from build123d import *

# Parameters (mm, degrees)
F0_W     = 63.5
F0_H     = 71.628
F1_DEPTH = 21.59
F2_W     = 36.83
F2_H     = 50.8
F3_DEPTH = 21.59
F5_DEPTH = 50.8
F6_R     = 3.937
F7_DEPTH = 43.181


with BuildPart() as f1:
    # F0 (on Top) → F1 (new body)
    with BuildSketch(Plane.XY):
        with Locations((31.75, 35.814)):
            Rectangle(F0_W, F0_H)
    extrude(amount=-F1_DEPTH)

    # F2 (on face) → F3 (join)
    with BuildSketch(Plane.XY):
        with Locations((28.575, 46.228)):
            Rectangle(F2_W, F2_H)
    extrude(amount=F3_DEPTH)

    # F4 (on face) → F5 (cut)
    with BuildSketch(Plane.XZ.offset(-20.828)):
        Polygon((10.16, 0), (16.51, 21.59), (10.16, 21.59), align=None)
    extrude(amount=-F5_DEPTH, mode=Mode.SUBTRACT)

    # F6 (on face) → F7 (cut, through all)
    with BuildSketch(Plane.XY.offset(21.59)):
        with Locations((31.54692, 43.815)):
            Circle(F6_R)
    extrude(amount=-F7_DEPTH, mode=Mode.SUBTRACT)


solid = f1.part
Verification items for the finished model (mm, model axes). A direction names the side the tool comes from. Round coordinates to 2 decimals unless told otherwise and drop trailing zeros. Write each loop counter-clockwise with the first axis right and the second up, starting at its lowest first coordinate (ties: lowest second). Pieces come first, ordered by that corner, then holes.
(1) Mould release check, pull along Y, two halves, no side actions. Record for faces 4 (the flat face through (31, 0, -11)), 5 (the cylindrical face through (27.614, 43.988, 0.302)), 6 (the flat face through (63.5, 35, -11)): pulls with the +Y half, pulls with the -Y half, needs draft (parallel to the pull), parting line crosses it, or undercut.
Returned:
face 4: pulls with the -Y half
face 5: undercut
face 6: needs draft
(2) Section check B-B (y = 30). Enter the section's corners in (x, z), plus the area to 3 significant figures.
Returned:
outline: (0, -21.59) - (63.5, -21.59) - (63.5, 0) - (46.99, 0) - (46.99, 21.59) - (16.51, 21.59) - (10.16, 0) - (0, 0) - close
area: 2,100 mm2
(3) Section check D-D (z = 11.5). Enter the section's corners in (x, y) (3 decimals).
Returned:
outline: (13.542, 20.828) - (46.99, 20.828) - (46.99, 71.628) - (13.542, 71.628) - close; hole circle Ø7.874 at (31.547, 43.815)
(4) Material ranges on line 1 (Y direction, x = 40, z = 7); line 2 (Z direction, x = 42.5, y = 9); line 3 (Y direction, x = 32, z = -10), recorded low to high.
Returned:
line 1: y = 20.83 to 71.63
line 2: z = -21.59 to 0
line 3: y = 0 to 39.9, 47.73 to 71.63
(5) Section check A-A (x = 34). Enter the section's corners in (y, z).
Returned:
outline: (0, -21.59) - (40.74, -21.59) - (40.74, 21.59) - (20.83, 21.59) - (20.83, 0) - (0, 0) - close; (46.89, -21.59) - (71.63, -21.59) - (71.63, 21.59) - (46.89, 21.59) - close
(6) Access from +Z, -Z, +X, -X, +Y, -Y to the whole of each face (thin tool, end or side, straight path). Record for faces 1 (the flat face through (46.99, 46, 11)), 2 (the flat face through (31, 71.628, -4)), 3 (the flat face through (28, 20.828, 11)).
Returned:
face 1: +Z, +X, +Y, -Y
face 2: +Z, -Z, +X, -X, +Y
face 3: +Z, +X, -X, -Y
(7) Depth check by flat-ended pin: pin 1 Ø6 at (y, z) = (36, 4.5) entering from -X; pin 2 Ø12.5 at (x, y) = (31.55, 43.82) entering from +Z; pin 3 Ø6.5 at (x, z) = (32, 10.5) entering from -Y; pin 4 Ø12 at (x, y) = (56, 53.5) entering from +Z. Enter the tip coordinate at first touch or a pass-through.
Returned:
pin 1: stops at x = 10.6
pin 2: stops at z = 21.59
pin 3: stops at y = 20.83
pin 4: stops at z = 0
(8) Section check C-C (x = 18). Enter the section's corners in (y, z).
Returned:
outline: (0, -21.59) - (71.63, -21.59) - (71.63, 21.59) - (20.83, 21.59) - (20.83, 0) - (0, 0) - close
